Read the model definition and answer for the solid it produces. Units are mm, in the model's axes. Face numbers are marked on the shaded views. A direction names the side the tool comes from. Coordinates: 2 decimals unless noted, no trailing zeros. Order: outer loops, then holes, each group sorted by start corner. A loop starts at its lowest first (then second) coordinate and runs counter-clockwise, first axis right, second up. Notation, with made-up numbers: (64, 21) -> (105, 21) arc R19 cw to (105, 25) -> close; hole circle Ø7 at (-20.5, 11). An arc over 180 degrees is marked (long way). Answer as a JSON object with one key per item and string values. Group by question number.
1) Section C-C on z = -7 is taken. Determine the outline of the cut face in (x, y), and give its area (3 significant figures).
2) Determine the mould class of the marked faces 3, 4 and 5 for opening direction X: released by +X, released by -X, zero draft, split by the parting line, or undercut.
3) Given pin 1 (2 mm diameter, centred on x = -12.5, z = -29.5, fed in from +Y); pin 2 (5 mm diameter, centred on x = -15, y = 11.5, fed in from -Z), each flat-ended and moving along its own axis, determine where each tip first touches the part or whether it passes through.
4) A tool of negligible diameter and unlimited length cuts with its end or side. For the marked faces 1 and 2, from which of +Z, -Z, +X, -X, +Y, -Y can it reach the whole face along a straight path? Write none if from no direction.
5) Consider L1, parallel to X at y = 12.25, z = -32; L2, parallel to Z at x = -20.5, y = 16; L3, parallel to X at y = 11.25, z = -12. Determine where each line is inside the solid, lowest interval first.
6) Section D-D on x = -18.75 is taken. Determine the outline of the cut face in (y, z).
7) Section B-B on y = 12.5 is taken. Determine the outline of the cut face in (x, z), and give its area (3 significant figures).
8) Section A-A on x = -22.5 is taken. Determine the outline of the cut face in (y, z).
Autodesk Inventor part; units mm, degrees
ref_plane "YZ Plane" through (0, 0, 0) normal (1, 0, 0) x (0, 1, 0)
ref_plane "XZ Plane" through (0, 0, 0) normal (0, 1, 0) x (-1, 0, 0)
ref_plane "XY Plane" through (0, 0, 0) normal (0, 0, 1) x (1, 0, 0)
sketch "Sketch1" plane through (0, 0, 0) normal (0, 0, 1) x (1, 0, 0)
  line L0 (-2.5, 7.5) -> (-27.5, 7.5)
  line L1 (-27.5, 7.5) -> (-27.5, 17.5)
  line L2 (-27.5, 17.5) -> (-2.5, 17.5)
  line L3 (-2.5, 17.5) -> (-2.5, 7.5)
  point P0 (0, 0)
  dimension "d0" = 10
  dimension "d1" = 25
  dimension "d2" = 2.5
  dimension "d3" = 7.5
extrude "Extrusion1" add sketch "Sketch1" along normal blind 20
sketch "Sketch2" plane through (0, 0, 20) normal (0, 0, 1) x (1, 0, 0)
  circle A0 centre (-7.5, 12.5) radius 2.25
  circle A1 centre (-22.5, 12.5) radius 2.25
  line L0 (-27.5, 7.5) -> (-2.5, 7.5)
  line L1 (-27.5, 17.5) -> (-27.5, 7.5)
  line L2 (-2.5, 7.5) -> (-2.5, 17.5)
  point P0 (0, 0)
  dimension "d6" = 4.5
  dimension "d7" = 5
  dimension "d8" = 5
  dimension "d9" = 5
  dimension "d10" = 5
extrude "Extrusion2" add sketch "Sketch2" against normal blind 60
properties part number "arm_safe"
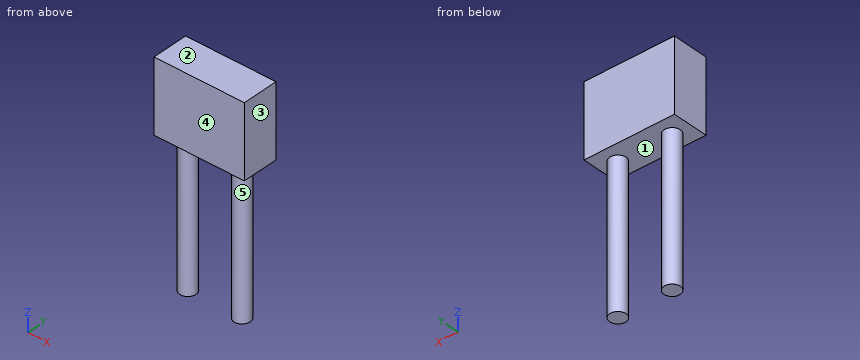
Worked answers:
{
 "1": {"outline": "circle Ø4.5 at (-22.5, 12.5); circle Ø4.5 at (-7.5, 12.5)", "area": "31.8 mm²"},
 "2": {"face 3": "released by +X", "face 4": "zero draft", "face 5": "undercut"},
 "3": {"pin 1": "passes through", "pin 2": "stops at z = 0"},
 "4": {"face 1": "-Z", "face 2": "+Z, +X, -X, +Y, -Y"},
 "5": {"L1": "x = -24.74 to -20.26, -9.74 to -5.26", "L2": "z = 0 to 20", "L3": "x = -24.37 to -20.63, -9.37 to -5.63"},
 "6": {"outline": "(7.5, 0) -> (17.5, 0) -> (17.5, 20) -> (7.5, 20) -> close"},
 "7": {"outline": "(-27.5, 0) -> (-24.75, 0) -> (-24.75, -40) -> (-20.25, -40) -> (-20.25, 0) -> (-9.75, 0) -> (-9.75, -40) -> (-5.25, -40) -> (-5.25, 0) -> (-2.5, 0) -> (-2.5, 20) -> (-27.5, 20) -> close", "area": "860 mm²"},
 "8": {"outline": "(7.5, 0) -> (10.25, 0) -> (10.25, -40) -> (14.75, -40) -> (14.75, 0) -> (17.5, 0) -> (17.5, 20) -> (7.5, 20) -> close"}
}
